```python
from build123d import *

# Parameters (mm, degrees)
F0_R     = 1.7272
F0_R_2   = 3.96875
F0_R_3   = 4.7625
F0_R_4   = 8.221183
F0_R_5   = 3.175
F1_DEPTH = 3.175


with BuildPart() as f1:
    # F0 (on Top) → F1 (new body)
    with BuildSketch(Plane.XY):
        with BuildLine():
            Line((-426.540354, 38.03015), (-488.352253, 21.467701))
            ThreePointArc((-488.352253, 21.467701), (-504.825, 0), (-488.352253, -21.467701))
            Line((-488.352253, -21.467701), (-426.540354, -38.03015))
            Line((-426.540354, -38.03015), (-420.190354, -38.03015))
            Line((-420.190354, -38.03015), (-62.409646, -38.03015))
            Line((-62.409646, -38.03015), (-56.059646, -38.03015))
            Line((-56.059646, -38.03015), (5.752253, -21.467701))
            ThreePointArc((5.752253, -21.467701), (22.225, 0), (5.752253, 21.467701))
            Line((5.752253, 21.467701), (-56.059646, 38.03015))
            Line((-56.059646, 38.03015), (-62.409646, 38.03015))
            Line((-62.409646, 38.03015), (-420.190354, 38.03015))
            Line((-420.190354, 38.03015), (-426.540354, 38.03015))
        make_face()
        with Locations((-405.902854, -30.09265)):
            Circle(F0_R, mode=Mode.SUBTRACT)
        with Locations((-494.386586, -11.786586)):
            Circle(F0_R, mode=Mode.SUBTRACT)
        with Locations((-470.813414, -11.786586)):
            Circle(F0_R_2, mode=Mode.SUBTRACT)
        with Locations((-76.697146, -30.09265)):
            Circle(F0_R, mode=Mode.SUBTRACT)
        with Locations((-11.786586, -11.786586)):
            Circle(F0_R_2, mode=Mode.SUBTRACT)
        with Locations((11.786586, -11.786586)):
            Circle(F0_R, mode=Mode.SUBTRACT)
        with Locations((-482.6, 0)):
            Circle(F0_R_3, mode=Mode.SUBTRACT)
        with Locations((-494.386586, 11.786586)):
            Circle(F0_R_2, mode=Mode.SUBTRACT)
        with Locations((-470.813414, 11.786586)):
            Circle(F0_R, mode=Mode.SUBTRACT)
        with Locations((-405.902854, 30.09265)):
            Circle(F0_R, mode=Mode.SUBTRACT)
        with Locations((-50.8, 0)):
            Circle(F0_R_4, mode=Mode.SUBTRACT)
        Circle(F0_R_5, mode=Mode.SUBTRACT)
        with Locations((-11.786586, 11.786586)):
            Circle(F0_R, mode=Mode.SUBTRACT)
        with Locations((11.786586, 11.786586)):
            Circle(F0_R_2, mode=Mode.SUBTRACT)
        with Locations((-76.697146, 30.09265)):
            Circle(F0_R, mode=Mode.SUBTRACT)
    extrude(amount=F1_DEPTH)


solid = f1.part
```
The model under review builds one solid part; all positions refer to its coordinate system, in mm. Round coordinates to 2 decimals unless told otherwise and drop trailing zeros. Loops run counter-clockwise (first coordinate to the right, second up) from the corner with the lowest first, then second, coordinate; pieces in that order, holes last. Notation, with made-up numbers: (44.5, 50) -> (70.5, 50) arc R26 ccw to (70.5, 68) -> close; hole circle Ø9 at (36.25, 2). An arc over 180 degrees is marked (long way). Answer as a JSON object with one key per item and string values. Group by question number.
1) For line 1 (X direction, y = 0.5, z = 0.85); line 2 (X direction, y = -12, z = 2.3); line 3 (X direction, y = -11, z = 3), list the stretches that pass through material, from the lowest coordinate up. Write a range as [from, to].
2) We need section B-B on z = 1.3. Give the number of separate pieces and of enclosed holes in the cut face, then the cut area to 3 significant figures.
3) We need section C-C on x = -482.6. Write out the cut boundary in (y, z) (1 decimal).
4) We need section A-A on x = -50.8. Write out the cut boundary in (y, z) (3 decimals).
5) Mouldability with a two-part tool opening along Y and no side actions: class faces 1 (the face through (-487.358, 0.209, 1.565)), 2 (the face through (-245, 1, 0)), 3 (the face through (-25.586, -29.865, 1.565)) as released by +Y, released by -Y, zero draft, split by the parting line, or undercut.
Result set:
{
 "1": {"line 1": "[-504.82, -487.34], [-477.86, -59.01], [-42.59, -3.14], [3.14, 22.22]", "line 2": "[-501.31, -496.1], [-492.67, -474.78], [-466.85, -15.75], [-7.82, 10.07], [13.5, 18.71]", "line 3": "[-501.91, -495.92], [-492.85, -474.7], [-466.92, -15.68], [-7.9, 10.25], [13.32, 19.31]"},
 "2": {"separate pieces": "1", "enclosed holes": "15", "area": "36,000 mm²"},
 "3": {"outline": "(-23, 0) -> (-4.8, 0) -> (-4.8, 3.2) -> (-23, 3.2) -> close; (4.8, 0) -> (23, 0) -> (23, 3.2) -> (4.8, 3.2) -> close"},
 "4": {"outline": "(-36.621, 0) -> (-8.221, 0) -> (-8.221, 3.175) -> (-36.621, 3.175) -> close; (8.221, 0) -> (36.621, 0) -> (36.621, 3.175) -> (8.221, 3.175) -> close"},
 "5": {"face 1": "undercut", "face 2": "zero draft", "face 3": "released by -Y"}
}
